from build123d import *

# Parameters (mm, degrees)
F1_DEPTH  = 16
F2_R      = 1.75
F3_DEPTH  = 25
F5_DEPTH  = 25
F6_R      = 2
F7_R      = 3
F8_R      = 1
F9_R      = 3
F9_R_2    = 1.75
F10_DEPTH = 2
F11_R     = 1


with BuildPart() as f1:
    # F0 (on Front) → F1 (new body)
    with BuildSketch(Plane.XZ):
        Polygon((0, 4.745212), (0, 0), (20, 0), (20, 19.745212), (30, 19.745212), (30, 22.745212), (15, 22.745212), (15, 4.745212), align=None)
    extrude(amount=F1_DEPTH)

    # F2 (on face) → F3 (cut)
    with BuildSketch(Plane.XY.offset(22.745212)):
        with Locations((25, -3)):
            Circle(F2_R)
        with Locations((25, -13)):
            Circle(F2_R)
    extrude(amount=-F3_DEPTH, mode=Mode.SUBTRACT)

    # F4 (on face) → F5 (cut)
    with BuildSketch(Plane.XY.offset(4.745212)):
        with BuildLine():
            ThreePointArc((3.031373, -7.5), (3, -8), (3.031373, -8.5))
            ThreePointArc((3.031373, -8.5), (9.828427, -10.828427), (7.5, -4.031373))
            ThreePointArc((7.5, -4.031373), (7, -4), (6.5, -4.031373))
            ThreePointArc((6.5, -4.031373), (4.171573, -5.171573), (3.031373, -7.5))
        make_face()
        with BuildLine():
            ThreePointArc((6.5, -4.031373), (7, -4), (7.5, -4.031373))
            Line((7.5, -4.031373), (7.5, 0.274567))
            Line((7.5, 0.274567), (6.5, 0.274567))
            Line((6.5, 0.274567), (6.5, -4.031373))
        make_face()
    extrude(amount=-F5_DEPTH, mode=Mode.SUBTRACT)

    # F6
    f6_edges = [f1.edges().sort_by_distance(p)[0] for p in [
        (15, -8, 4.745212),
    ]]
    fillet(f6_edges, radius=F6_R)

    # F7
    f7_edges = [f1.edges().sort_by_distance(p)[0] for p in [
        (15, -8, 22.745212),
    ]]
    fillet(f7_edges, radius=F7_R)

    # F8
    f8_edges = [f1.edges().sort_by_distance(p)[0] for p in [
        (30, -8, 22.745212),
        (24, -16, 22.745212),
        (24, 0, 22.745212),
    ]]
    fillet(f8_edges, radius=F8_R)

    # F9 (on face) → F10 (join)
    with BuildSketch(Plane.XY.offset(22.745212)):
        with Locations((25, -3)):
            Circle(F9_R)
        with Locations((25, -3)):
            Circle(F9_R_2, mode=Mode.SUBTRACT)
        with Locations((25, -13)):
            Circle(F9_R)
        with Locations((25, -13)):
            Circle(F9_R_2, mode=Mode.SUBTRACT)
    extrude(amount=-F10_DEPTH)

    # F11
    f11_edges = [f1.edges().sort_by_distance(p)[0] for p in [
        (3.25, 0, 4.745212),
    ]]
    fillet(f11_edges, radius=F11_R)


solid = f1.part
Could you check a few things on this model? Use its own coordinates, in mm. A direction names the side the tool comes from. Give positions to 0.01 mm unless a question says otherwise; leave off trailing zeros. Order: outer loops, then holes, each group sorted by start corner. A loop starts at its lowest first (then second) coordinate and runs counter-clockwise, first axis right, second up. Notation, with made-up numbers: (-3.5, 23) - (45.5, 23) arc R12 ccw to (45.5, 33) - close; hole circle Ø1 at (47, 41.25). An arc over 180 degrees is marked (long way). Return JSON: item names as keys, results as strings. Group by question number.
Q1. Suppose I cut it at D-D, the plane z = 12. Please give me the cut outline in (x, y), and give its area (3 significant figures).
Q2. Which directions (+Z, -Z, +X, -X, +Y, -Y) give clear straight access to the entire face, cutting with the end or side of a thin tool? Please do faces 5 (the face through (6.41, -15.7, 4.46)), 6 (the face through (25, -16, 22)), 7 (the face through (15, -8, 13)), 8 (the face through (25, 0, 22)).
Q3. Thinking about a two-plate mould opening in Y: for faces 1 (the face through (7.5, -2, 2)), 2 (the face through (15.285, -15.699, 13.154)), 3 (the face through (23.71, -11.82, 21.27)), 4 (the face through (10.212, -0.285, 4.445)), which applies, pulls with the +Y half, pulls with the -Y half, needs draft (parallel to the pull), parting line crosses it, or undercut?
Q4. Will these pins go through, and if not, where does the flat tip stop? pin 1 Ø6.5 at (x, y) = (6, -10.5) entering from +Z; pin 2 Ø6.5 at (y, z) = (-7, 10.5) entering from -X; pin 3 Ø10 at (x, z) = (4, 13.5) entering from -Y; pin 4 Ø3 at (y, z) = (-2, 1.5) entering from +X.
Q5. Please list where these lines run through material, in increasing order: line 1 along Y through (x, z) = (25, 20.3); line 2 along X through (y, z) = (-8, 2.1); line 3 along X through (y, z) = (-3.25, 1.75). Write a range as [from, to].
Q6. Suppose I cut it at A-A, the plane y = -3. Please give me the cut outline in (x, z), and give its area (3 significant figures).
Q7. Suppose I cut it at C-C, the plane x = 10. Please give me the cut outline in (y, z).
Q8. Suppose I cut it at B-B, the plane y = -13. Please give me the cut outline in (x, z), and give its area (3 significant figures).
Resolved:
{
 "1": {"outline": "(15, -15) arc R1 ccw to (16, -16) - (20, -16) - (20, 0) - (16, 0) arc R1 ccw to (15, -1) - close", "area": "79.6 mm2"},
 "2": {"face 5": "+Z, -X, -Y", "face 6": "+Z, -Y", "face 7": "+Z, -X, +Y, -Y", "face 8": "+Z, +Y"},
 "3": {"face 1": "needs draft", "face 2": "pulls with the -Y half", "face 3": "undercut", "face 4": "pulls with the +Y half"},
 "4": {"pin 1": "stops at z = 4.75", "pin 2": "stops at x = 15", "pin 3": "passes through", "pin 4": "stops at x = 20"},
 "5": {"line 1": "y = [-16, -14.75], [-11.25, -4.75], [-1.25, 0]", "line 2": "x = [0, 3], [11, 20]", "line 3": "x = [0, 6.5], [7.5, 20]"},
 "6": {"outline": "(0, 0) - (6.5, 0) - (6.5, 4.75) - (0, 4.75) - close; (7.5, 0) - (20, 0) - (20, 19.75) - (23.25, 19.75) - (23.25, 22.75) - (18, 22.75) arc R3 ccw to (15, 19.75) - (15, 6.75) arc R2 cw to (13, 4.75) - (7.5, 4.75) - close; (26.75, 19.75) - (30, 19.75) - (30, 21.75) arc R1 ccw to (29, 22.75) - (26.75, 22.75) - close", "area": "198 mm2"},
 "7": {"outline": "(-16, 0) - (-10.65, 0) - (-10.65, 4.75) - (-15, 4.75) arc R1 ccw to (-16, 3.75) - close; (-5.35, 0) - (0, 0) - (0, 3.75) arc R1 ccw to (-1, 4.75) - (-5.35, 4.75) - close"},
 "8": {"outline": "(0, 0) - (20, 0) - (20, 19.75) - (23.25, 19.75) - (23.25, 22.75) - (18, 22.75) arc R3 ccw to (15, 19.75) - (15, 6.75) arc R2 cw to (13, 4.75) - (0, 4.75) - close; (26.75, 19.75) - (30, 19.75) - (30, 21.75) arc R1 ccw to (29, 22.75) - (26.75, 22.75) - close", "area": "203 mm2"}
}
